from build123d import *

# Parameters (mm, degrees)
BOSS_EXTRUDE1_DEPTH = 12
FILLET1_R           = 3
BOSS_EXTRUDE2_DEPTH = 5
FILLET2_R           = 2
SKETCH4_R           = 1.75
BOSS_EXTRUDE3_DEPTH = 10
SKETCH5_R           = 2
BOSS_EXTRUDE4_DEPTH = 10
FILLET3_R           = 2


with BuildPart() as part:
    # Sketch1 → Boss-Extrude1 (new body)
    with BuildSketch(Plane(origin=(0, 0, 0), x_dir=(1, 0, 0), z_dir=(0, 1, 0))):
        Polygon((-6, 0), (6, 0), (11, 17), (16, 34), (16, 46), (-16, 46), (-16, 34), (-11, 17), align=None)
    extrude(amount=BOSS_EXTRUDE1_DEPTH)

    # Fillet1
    fillet1_edges = [part.edges().sort_by_distance(p)[0] for p in [
        (11, 12, -17),
        (16, 12, -40),
        (-16, 12, -40),
        (-11, 12, -17),
        (-11, 0, -17),
        (-16, 0, -40),
        (16, 0, -40),
        (11, 0, -17),
    ]]
    fillet(fillet1_edges, radius=FILLET1_R)

    # Sketch3 → Boss-Extrude2 (add)
    with BuildSketch(Plane(origin=(0, 0, -46), x_dir=(-1, 0, 0), z_dir=(0, 0, -1))):
        Polygon((-13, 13), (13, 13), (20, 6), (13, -1), (-13, -1), (-20, 6), align=None)
    extrude(amount=BOSS_EXTRUDE2_DEPTH)

    # Fillet2
    fillet2_edges = [part.edges().sort_by_distance(p)[0] for p in [
        (13, 13, -48.5),
        (20, 6, -48.5),
        (13, -1, -48.5),
        (-13, -1, -48.5),
        (-20, 6, -48.5),
        (-13, 13, -48.5),
    ]]
    fillet(fillet2_edges, radius=FILLET2_R)

    # Sketch4 → Boss-Extrude3 (add)
    with BuildSketch(Plane(origin=(0, 0, -51), x_dir=(-1, 0, 0), z_dir=(0, 0, -1))):
        with Locations((-10, 6)):
            Circle(SKETCH4_R)
        with Locations((10, 6)):
            Circle(SKETCH4_R)
    extrude(amount=BOSS_EXTRUDE3_DEPTH)

    # Sketch5 → Boss-Extrude4 (add)
    with BuildSketch(Plane(origin=(0, 0, -61), x_dir=(-1, 0, 0), z_dir=(0, 0, -1))):
        with Locations((10, 6)):
            Circle(SKETCH5_R)
        with Locations((-10, 6)):
            Circle(SKETCH5_R)
    extrude(amount=BOSS_EXTRUDE4_DEPTH)

    # Fillet3
    fillet3_edges = [part.edges().sort_by_distance(p)[0] for p in [
        (-8, 6, -71),
        (12, 6, -71),
    ]]
    fillet(fillet3_edges, radius=FILLET3_R)


solid = part.part
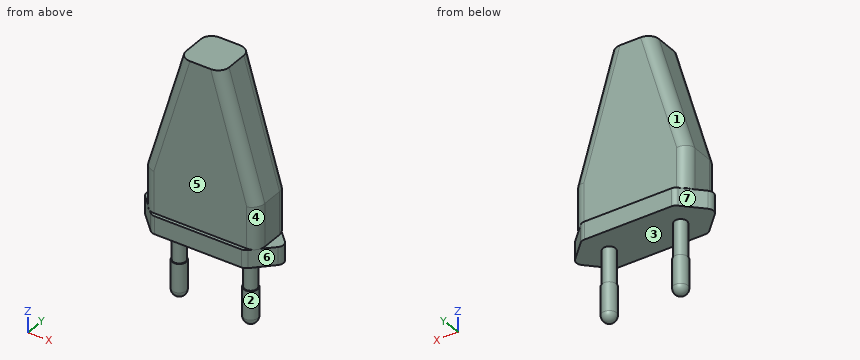
For this review, take the finished solid that the model builds, in its own axes (mm). Face numbers are marked on the shaded views. A direction names the side the tool comes from. Round coordinates to 2 decimals unless told otherwise and drop trailing zeros. Loops run counter-clockwise (first coordinate to the right, second up) from the corner with the lowest first, then second, coordinate; pieces in that order, holes last. Notation, with made-up numbers: (-34, 48.5) - (-18, 48.5) arc R20 cw to (-18, 59.5) - close; hole circle Ø6 at (76, 84.5). An arc over 180 degrees is marked (long way). One line per item, written item: value. Start each with the question number.
Item 1: Take a section at A-A (x = 0.5). Give the boundary of the cut face in (y, z), plus the area to 3 significant figures.
Item 2: Take a section at D-D (z = -44.5). Give the boundary of the cut face in (x, y), plus the area to 3 significant figures.
Item 3: For the marked faces 5, 6 and 7, list the 3-axis set-ups (+Z, -Z, +X, -X, +Y, -Y) from which the entire face can be reached by the end or side of a thin tool; tool diameter is ignored.
Item 4: For L1, parallel to Y at x = -1, z = -34.5; L2, parallel to X at y = 4, z = -44; L3, parallel to Z at x = -3.5, y = 1.5, list the stretches that pass through material, from the lowest coordinate up.
Item 5: The part is to be moulded in two halves that separate along X. For the marked faces 1, 2, 3 and 4, say which applies: +X half, -X half, draft (parallel to the pull), parting line (faces both ways), or undercut.
Item 6: Clearance check with flat-ended pins moving along their axes: pin 1 Ø12 at (x, z) = (1, -27) entering from -Y; pin 2 Ø0.7 at (x, y) = (-15, 1) entering from -Z; pin 3 Ø5 at (y, z) = (1, -25) entering from -X. State where each tip first meets the part, or that it passes through.
Item 7: Take a section at B-B (z = -53.5). Give the boundary of the cut face in (x, y), plus the area to 3 significant figures.
Item 8: Take a section at C-C (y = 6). Give the boundary of the cut face in (x, z), plus the area to 3 significant figures.
Answer below:
1. outline: (-1, -51) - (13, -51) - (13, -46) - (12, -46) - (12, 0) - (0, 0) - (0, -46) - (-1, -46) - close
1. area: 622 mm2
2. outline: (-16, 3) arc R3 ccw to (-13, 0) - (13, 0) arc R3 ccw to (16, 3) - (16, 9) arc R3 ccw to (13, 12) - (-13, 12) arc R3 ccw to (-16, 9) - close
2. area: 376 mm2
3. face 5: +Z, +X, -X, -Y
3. face 6: -Z, +X, -Y
3. face 7: -Z, -X, +Y
4. L1: y = 0 to 12
4. L2: x = -16 to 16
4. L3: z = -51 to 0
5. face 1: -X half
5. face 2: undercut
5. face 3: undercut
5. face 4: +X half
6. pin 1: stops at y = 0
6. pin 2: stops at z = -51
6. pin 3: stops at x = -13.9
7. outline: circle Ø3.5 at (-10, 6); circle Ø3.5 at (10, 6)
7. area: 19.2 mm2
8. outline: (-19.17, -51) - (-11.75, -51) - (-11.75, -61) - (-12, -61) - (-12, -69) arc R2 ccw to (-8, -69) - (-8, -61) - (-8.25, -61) - (-8.25, -51) - (8.25, -51) - (8.25, -61) - (8, -61) - (8, -69) arc R2 ccw to (12, -69) - (12, -61) - (11.75, -61) - (11.75, -51) - (19.17, -51) - (19.17, -46) - (16, -46) - (16, -34) - (6, 0) - (-6, 0) - (-16, -34) - (-16, -46) - (-19.17, -46) - close
8. area: 1,470 mm2
